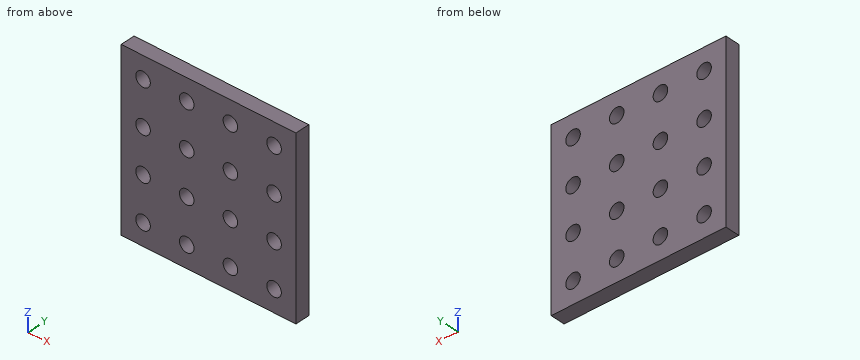
from build123d import *

# Parameters (mm, degrees)
SKETCH1_W            = 120
SKETCH1_H            = 120
BOSS_EXTRUDE1_DEPTH  = 10
SKETCH2_R            = 5
CUT_EXTRUDE1_DEPTH   = 11
LPATTERN1_COUNT      = 4
LPATTERN1_PITCH      = 30
LPATTERN1_COUNT_DIR2 = 4
LPATTERN1_PITCH_DIR2 = 30


with BuildPart() as part:
    # Sketch1 → Boss-Extrude1 (new body)
    with BuildSketch(Plane(origin=(0, 0, 0), x_dir=(1, 0, 0), z_dir=(0, 1, 0))):
        with Locations((60, 60)):
            Rectangle(SKETCH1_W, SKETCH1_H)
    extrude(amount=BOSS_EXTRUDE1_DEPTH)

    # Sketch2 → Cut-Extrude1 (cut, through all)
    with BuildSketch(Plane(origin=(0, 10, 0), x_dir=(1, 0, 0), z_dir=(0, 1, 0))):
        with Locations((15, 15)):
            Circle(SKETCH2_R)
    cut_extrude1 = extrude(amount=-CUT_EXTRUDE1_DEPTH, mode=Mode.SUBTRACT)

    # LPattern1: Cut-Extrude1 4 × 4
    with Locations(*[(i * LPATTERN1_PITCH, 0, -j * LPATTERN1_PITCH_DIR2) for i in range(LPATTERN1_COUNT) for j in range(LPATTERN1_COUNT_DIR2) if (i, j) != (0, 0)]):
        add(cut_extrude1, mode=Mode.SUBTRACT)


solid = part.part
The listing builds one solid part. Answer for the finished solid, in the listing's coordinates (mm). Give positions to 0.01 mm unless a question says otherwise; leave off trailing zeros. Order: outer loops, then holes, each group sorted by start corner. A loop starts at its lowest first (then second) coordinate and runs counter-clockwise, first axis right, second up. Notation, with made-up numbers: (0, 21) - (35, 21) arc R32 cw to (35, 52) - close; hole circle Ø3 at (54, 5.25). An arc over 180 degrees is marked (long way). One line per item, written item: value. Start each with the question number.
1) A cutting plane is placed at A-A on z = -15. Give the vertices of the cut face in (x, y), then the cut area to 3 significant figures.
2) Given pin 1 Ø16 at (x, z) = (45, -105) entering from -Y, flat-ended and moving along its own axis, determine where the tip first touches the part or whether it passes through.
3) Find the intervals of material crossed by L1, parallel to X at y = 4, z = -75; L2, parallel to Z at x = 45, y = 2; L3, parallel to X at y = 2.25, z = -16.5, in increasing order.
4) A cutting plane is placed at B-B on x = 45. Give the vertices of the cut face in (y, z), then the cut area to 3 significant figures.
5) A cutting plane is placed at C-C on y = 3.75. State how many separate pieces and enclosed holes the cut face has, then the cut area to 3 significant figures.
Answer sheet:
1. outline: (0, 0) - (10, 0) - (10, 10) - (0, 10) - close; (20, 0) - (40, 0) - (40, 10) - (20, 10) - close; (50, 0) - (70, 0) - (70, 10) - (50, 10) - close; (80, 0) - (100, 0) - (100, 10) - (80, 10) - close; (110, 0) - (120, 0) - (120, 10) - (110, 10) - close
1. area: 800 mm2
2. pin 1: stops at y = 0
3. L1: x = 0 to 10, 20 to 40, 50 to 70, 80 to 100, 110 to 120
3. L2: z = -120 to -110, -100 to -80, -70 to -50, -40 to -20, -10 to 0
3. L3: x = 0 to 10.23, 19.77 to 40.23, 49.77 to 70.23, 79.77 to 100.23, 109.77 to 120
4. outline: (0, -120) - (10, -120) - (10, -110) - (0, -110) - close; (0, -100) - (10, -100) - (10, -80) - (0, -80) - close; (0, -70) - (10, -70) - (10, -50) - (0, -50) - close; (0, -40) - (10, -40) - (10, -20) - (0, -20) - close; (0, -10) - (10, -10) - (10, 0) - (0, 0) - close
4. area: 800 mm2
5. separate pieces: 1
5. enclosed holes: 16
5. area: 13,100 mm2
